```python
from build123d import *

# Parameters (mm, degrees)
BOSS_EXTRUDE1_DEPTH = 17
CUT_EXTRUDE1_DEPTH  = 7


with BuildPart() as part:
    # Sketch1 → Revolve1 (revolve)
    with BuildSketch(Plane.XY, mode=Mode.PRIVATE) as revolve1_sk:
        with BuildLine():
            ThreePointArc((31.477739174, 1.289033786), (44.553939615, 13.368129979), (50.9, 30))
            Line((50.9, 30), (50.9, 0))
            Line((50.9, 0), (50.9, -7))
            Line((50.9, -7), (50.9, -27))
            Line((50.9, -27), (47.9, -27))
            Line((47.9, -27), (47.9, -7))
            Line((47.9, -7), (0, -7))
            Line((0, -7), (0, 0))
            Line((0, 0), (0, 15))
            ThreePointArc((0, 15), (15.444355802, 12.116315948), (27.574800041, 2.13152339))
            ThreePointArc((27.574800041, 2.13152339), (29.365754755, 0.96667333), (31.477739174, 1.289033786))
        make_face()
    revolve(revolve1_sk.sketch.rotate(Axis((0, 0, 0), (0, 1, 0)), 90), axis=Axis((0, 0, 0), (0, 1, 0)))

    # Sketch2 → Boss-Extrude1 (add)
    with BuildSketch(Plane.XZ.offset(7)):
        with BuildLine():
            Line((7.764571353, -28.977774789), (9.576304669, -35.739255573))
            ThreePointArc((9.576304669, -35.739255573), (0, -37), (-9.576304669, -35.739255573))
            Line((-9.576304669, -35.739255573), (-7.764571353, -28.977774789))
            ThreePointArc((-7.764571353, -28.977774789), (0, -30), (7.764571353, -28.977774789))
        make_face()
        with BuildLine():
            Line((28.977774789, 7.764571353), (35.739255573, 9.576304669))
            ThreePointArc((35.739255573, 9.576304669), (37, 0), (35.739255573, -9.576304669))
            Line((35.739255573, -9.576304669), (28.977774789, -7.764571353))
            ThreePointArc((28.977774789, -7.764571353), (30, 0), (28.977774789, 7.764571353))
        make_face()
        with BuildLine():
            Line((-28.977774789, -7.764571353), (-35.739255573, -9.576304669))
            ThreePointArc((-35.739255573, -9.576304669), (-37, 0), (-35.739255573, 9.576304669))
            Line((-35.739255573, 9.576304669), (-28.977774789, 7.764571353))
            ThreePointArc((-28.977774789, 7.764571353), (-30, 0), (-28.977774789, -7.764571353))
        make_face()
        with BuildLine():
            Line((-7.764571353, 28.977774789), (-9.576304669, 35.739255573))
            ThreePointArc((-9.576304669, 35.739255573), (0, 37), (9.576304669, 35.739255573))
            Line((9.576304669, 35.739255573), (7.764571353, 28.977774789))
            ThreePointArc((7.764571353, 28.977774789), (0, 30), (-7.764571353, 28.977774789))
        make_face()
    extrude(amount=BOSS_EXTRUDE1_DEPTH)

    # Sketch3 → Cut-Extrude1 (cut)
    with BuildSketch(Plane(origin=(0, -12, 0), x_dir=(-1, 0, 0), z_dir=(0, -1, 0))):
        with BuildLine():
            Line((3.777949646, -30.768930701), (4.387296363, -35.731661459))
            ThreePointArc((4.387296363, -35.731661459), (-2.511233055, -35.912305809), (-9.317485624, -34.773329746))
            Line((-9.317485624, -34.773329746), (-8.023390398, -29.943700615))
            ThreePointArc((-8.023390398, -29.943700615), (-2.162450686, -30.924485558), (3.777949646, -30.768930701))
        make_face()
        with BuildLine():
            Line((30.768930701, 3.777949646), (35.731661459, 4.387296363))
            ThreePointArc((35.731661459, 4.387296363), (35.912305809, -2.511233055), (34.773329746, -9.317485624))
            Line((34.773329746, -9.317485624), (29.943700615, -8.023390398))
            ThreePointArc((29.943700615, -8.023390398), (30.924485558, -2.162450686), (30.768930701, 3.777949646))
        make_face()
        with BuildLine():
            Line((-30.768930701, -3.777949646), (-35.731661459, -4.387296363))
            ThreePointArc((-35.731661459, -4.387296363), (-35.912305809, 2.511233055), (-34.773329746, 9.317485624))
            Line((-34.773329746, 9.317485624), (-29.943700615, 8.023390398))
            ThreePointArc((-29.943700615, 8.023390398), (-30.924485558, 2.162450686), (-30.768930701, -3.777949646))
        make_face()
        with BuildLine():
            Line((-3.777949646, 30.768930701), (-4.387296363, 35.731661459))
            ThreePointArc((-4.387296363, 35.731661459), (2.511233055, 35.912305809), (9.317485624, 34.773329746))
            Line((9.317485624, 34.773329746), (8.023390398, 29.943700615))
            ThreePointArc((8.023390398, 29.943700615), (2.162450686, 30.924485558), (-3.777949646, 30.768930701))
        make_face()
    extrude(amount=CUT_EXTRUDE1_DEPTH, mode=Mode.SUBTRACT)


solid = part.part
```
CAD build for the part. Positions are in the model's coordinates, mm. A direction names the side the tool comes from. Round coordinates to 2 decimals unless told otherwise and drop trailing zeros. Return JSON: item names as keys, results as strings. Group by question number.
Item 1: 3-axis set-ups, long thin cutter, end or side, ignore diameter. For faces 1 (the face through (2, -12, 33)), 2 (the face through (-7.878, -15.381, -29.401)): which of +Z, -Z, +X, -X, +Y, -Y reach the whole face in a straight line?
Item 2: Flat gauge pins, fed straight in: pin 1 Ø5 at (x, z) = (-4.5, -34.5) entering from -Y; pin 2 Ø3 at (x, z) = (32, -4) entering from +Y; pin 3 Ø10 at (x, y) = (36, -18.5) entering from +Z. Where does each tip first touch, or does it go through?
Item 3: Probe probe 1 along Z at (x, y) = (32.5, -20.5); probe 2 along X at (y, z) = (6.5, -18); probe 3 along Z at (x, y) = (23, 2). List the from-to ranges inside material, lowest first.
Item 4: Band-saw the part on A-A on y = -15. State how many separate pieces and enclosed holes the cut face has, plus the area to 3 significant figures.
Item 5: Mould opens along Z. For faces 3 (the face through (-33, -12, 2)), 4 (the face through (34, -27, 34)) say: +Z half, -Z half, draft (parallel to the pull), parting line (faces both ways), or undercut.
Resolved:
{
 "1": {"face 1": "none", "face 2": "-Y"},
 "2": {"pin 1": "stops at y = -24", "pin 2": "stops at y = 2.68", "pin 3": "stops at z = 40.37"},
 "3": {"probe 1": "z = -39.17 to -35.19, -8.71 to 8.71, 35.19 to 39.17", "probe 2": "x = -47.61 to -34.19, -15.45 to 15.45, 34.19 to 47.61", "probe 3": "z = -45.41 to -23.22, -15.39 to 15.39, 23.22 to 45.41"},
 "4": {"separate pieces": "5", "enclosed holes": "1", "area": "1,170 mm²"},
 "5": {"face 3": "undercut", "face 4": "draft"}
}
